Input: part model. Units: mm. Frame: model coordinates. Face numbers are marked on the shaded views. A direction names the side the tool comes from. Coordinates: 2 decimals unless noted, no trailing zeros. Write each loop counter-clockwise with the first axis right and the second up, starting at its lowest first coordinate (ties: lowest second). Pieces come first, ordered by that corner, then holes. Notation, with made-up numbers: M 27.5,72 L 75.5,72 A13 ccw 75.5,95 Z; hole C 3.5,-33.5 d9. An arc over 180 degrees is marked long. Use one line per item in the form item = value.
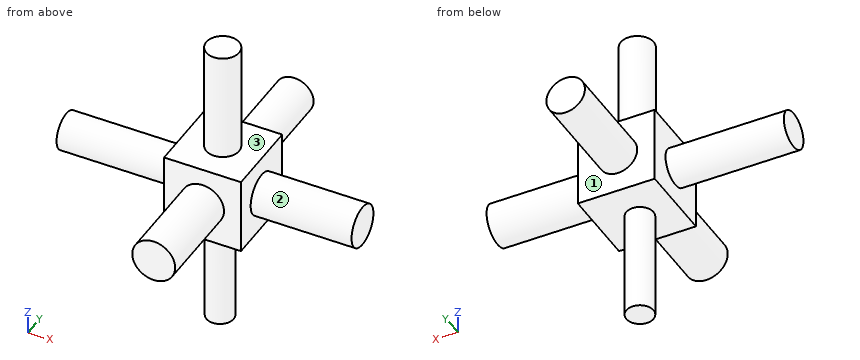
from build123d import *

# Parameters (mm, degrees)
F0_W      = 25
F0_H      = 25
F1_DEPTH  = 25.4
F2_R      = 5.34833
F3_DEPTH  = 60.688041
F5_R      = 4.425329
F6_DEPTH  = 35.64737
F4_R      = 5.771368
F7_DEPTH  = 5.648091
F8_R      = 6.258089
F9_DEPTH  = 32.231893
F10_R     = 6.97949
F11_DEPTH = 30.076189
F12_R     = 6.737557
F13_DEPTH = 32.785647
F14_R     = 6.042728
F15_DEPTH = 38.435884


with BuildPart() as f1:
    # F0 (on Front) → F1 (new body)
    with BuildSketch(Plane.XZ):
        with Locations((12.5, 12.5)):
            Rectangle(F0_W, F0_H)
    extrude(amount=F1_DEPTH)

    # F2 (on Top) → F3 (join)
    with BuildSketch(Plane.XY):
        with Locations((12.327284, -12.637898)):
            Circle(F2_R)
    extrude(amount=F3_DEPTH)

    # F5 (on face) → F6 (join)
    with BuildSketch(Plane(origin=(0, 0, 0), x_dir=(1, 0, 0), z_dir=(0, 0, -1))):
        with Locations((12.036352, 13.710335)):
            Circle(F5_R)
    extrude(amount=F6_DEPTH)

    # F4 (on Top) → F7 (join)
    with BuildSketch(Plane.XY):
        with Locations((11.907944, -12.260992)):
            Circle(F4_R)
    extrude(amount=F7_DEPTH)

    # F8 (on face) → F9 (join)
    with BuildSketch(Plane.XZ):
        with Locations((11.928667, 12.61479)):
            Circle(F8_R)
    extrude(amount=-F9_DEPTH)

    # F10 (on face) → F11 (join)
    with BuildSketch(Plane.XZ.offset(25.4)):
        with Locations((12.5, 12.5)):
            Circle(F10_R)
    extrude(amount=F11_DEPTH)

    # F12 (on face) → F13 (join)
    with BuildSketch(Plane.YZ.offset(25)):
        with Locations((-12.7, 12.28429)):
            Circle(F12_R)
    extrude(amount=F13_DEPTH)

    # F14 (on face) → F15 (join)
    with BuildSketch(Plane(origin=(0, 0, 0), x_dir=(0, -1, 0), z_dir=(-1, 0, 0))):
        with Locations((12.726512, 12.5)):
            Circle(F14_R)
    extrude(amount=F15_DEPTH)


solid = f1.part
(1) Line query: probe 1 along Y at (x, z) = (21.5, 2); probe 2 along Z at (x, y) = (22, -19); probe 3 along Y at (x, z) = (12, 25.5). Output: solid intervals per line, ascending.
Computed:
probe_1 = -25.4 to 0
probe_2 = 0 to 25
probe_3 = -17.98 to -7.3
(2) First-contact query: pin 1 Ø1.5 at (x, y) = (-25.5, -11) entering from +Z; pin 2 Ø12 at (x, z) = (-14.5, 5) entering from +Y; pin 3 Ø10 at (x, y) = (2.5, -40.5) entering from -Z. Flat tips, straight axial feed; report the tip coordinate or a pass-through.
Computed:
pin_1 = 18.46
pin_2 = -6.87
pin_3 = 7.63
(3) Section query B-B on x = 12.5. Return the cut outline in (y, z).
Computed:
outline = M -55.48,5.52 L -25.4,5.52 L -25.4,0 L -18.11,0 L -18.11,-35.65 L -9.31,-35.65 L -9.31,0 L 0,0 L 0,6.38 L 32.23,6.38 L 32.23,18.85 L 0,18.85 L 0,25 L -7.29,25 L -7.29,60.69 L -17.98,60.69 L -17.98,25 L -25.4,25 L -25.4,19.48 L -55.48,19.48 Z
(4) Section query A-A on z = 8.5. Return the cut outline in (x, y), plus the area to 3 significant figures.
Computed:
outline = M -38.44,-17.26 L 0,-17.26 L 0,-25.4 L 6.78,-25.4 L 6.78,-55.48 L 18.22,-55.48 L 18.22,-25.4 L 25,-25.4 L 25,-18.27 L 57.79,-18.27 L 57.79,-7.13 L 25,-7.13 L 25,0 L 16.64,0 L 16.64,32.23 L 7.21,32.23 L 7.21,0 L 0,0 L 0,-8.2 L -38.44,-8.2 Z
area = 2,000 mm^2
(5) Section query D-D on z = 54.5. Return the cut outline in (x, y), plus the area to 3 significant figures.
Computed:
outline = C 12.33,-12.64 d10.7
area = 89.9 mm^2
(6) Section query C-C on y = -37. Return the cut outline in (x, z), plus the area to 3 significant figures.
Computed:
outline = C 12.5,12.5 d13.96
area = 153 mm^2
(7) Set-up query: the marked faces 1, 2 and 3. Return all of +Z, -Z, +X, -X, +Y, -Y with unobstructed straight access to the full face (end or side cutting, diameter ignored); none if empty.
Computed:
face_1 = +Y
face_2 = +X
face_3 = +Z
